The listing builds one solid part. Answer for the finished solid, in the listing's coordinates (mm). A direction names the side the tool comes from. Coordinates: 2 decimals unless noted, no trailing zeros. Loops run counter-clockwise (first coordinate to the right, second up) from the corner with the lowest first, then second, coordinate; pieces in that order, holes last. Notation, with made-up numbers: M 86.5,59.25 L 124.5,59.25 A36 ccw 124.5,95.25 Z; hole C 57,-15 d4. An arc over 180 degrees is marked long. Return JSON: item names as keys, results as strings. Group by question number.
1. Section B-B (z = 282.5) is taken. Write down the section's boundary in (x, y).
2. Which of the six approach directions +Z, -Z, +X, -X, +Y, -Y give full straight-line access (tool end or side, diameter ignored) to faces 5 (the face through (11.5, 0, 222)), 6 (the face through (-1, -7, 0))?
3. Section A-A (y = 1.75) is taken. Write down the section's boundary in (x, z).
4. Straight lines are drawn through the part: L1, parallel to Y at x = -3.5, z = 142; L2, parallel to X at y = 7.3, z = 411.9; L3, parallel to X at y = -0.75, z = 75. For each, find the intervals that lie inside material, in ascending order. Write a range as from..to.
5. The mould has two halves that part along Y. Classify faces 1 (the face through (0, 6.5, 222)), 2 (the face through (-11.5, 0, 222)), 3 (the face through (0, 7.5, 222)), 4 (the face through (-1, -7, 450)): pulls with the +Y half, pulls with the -Y half, needs draft (parallel to the pull), parting line crosses it, or undercut.
```python
from build123d import *

# Parameters (mm, degrees)
SKETCH_1_W          = 25
SKETCH_1_H          = 15
SKETCH_1_W_2        = 23
SKETCH_1_H_2        = 13
EXTRUDE_1_DEPTH     = 450
SKETCH_2_R          = 2.6
CUT_EXTRUDE_1_DEPTH = 451.423411914


with BuildPart() as part:
    # ｽｹｯﾁ1 → ﾎﾞｽ - 押し出し1 (new body)
    with BuildSketch(Plane.XY):
        Rectangle(SKETCH_1_W, SKETCH_1_H)
        Rectangle(SKETCH_1_W_2, SKETCH_1_H_2, mode=Mode.SUBTRACT)
    extrude(amount=EXTRUDE_1_DEPTH)

    # ｽｹｯﾁ2 → ｶｯﾄ - 押し出し1 (cut, through all)
    with BuildSketch(Plane(origin=(0, 7.5, 0), x_dir=(1, 0, 0), z_dir=(0, 1, 0))):
        with Locations(Location((0, -12.7, 0), (0, 0, 270))):
            Circle(SKETCH_2_R)
        with Locations(Location((0, -25.4, 0), (0, 0, 270))):
            Circle(SKETCH_2_R)
        with Locations(Location((0, -38.1, 0), (0, 0, 270))):
            Circle(SKETCH_2_R)
    cut_extrude_1 = extrude(amount=-CUT_EXTRUDE_1_DEPTH, mode=Mode.SUBTRACT)

    # ﾐﾗｰ1: ｶｯﾄ - 押し出し1 across plane
    add(cut_extrude_1.mirror(Plane(origin=(0, 0, 225), x_dir=(1, 0, 0), z_dir=(0, 0, -1))), mode=Mode.SUBTRACT)


solid = part.part
```
Worked out:
{
 "1": {"outline": "M -12.5,-7.5 L 12.5,-7.5 L 12.5,7.5 L -12.5,7.5 Z; hole M -11.5,-6.5 L 11.5,-6.5 L 11.5,6.5 L -11.5,6.5 Z"},
 "2": {"face 5": "+Z, -Z", "face 6": "-Z, +X, -X, +Y, -Y"},
 "3": {"outline": "M -12.5,0 L -11.5,0 L -11.5,450 L -12.5,450 Z; M 11.5,0 L 12.5,0 L 12.5,450 L 11.5,450 Z"},
 "4": {"L1": "-7.5..-6.5, 6.5..7.5", "L2": "-12.5..-2.6, 2.6..12.5", "L3": "-12.5..-11.5, 11.5..12.5"},
 "5": {"face 1": "undercut", "face 2": "undercut", "face 3": "pulls with the +Y half", "face 4": "needs draft"}
}
